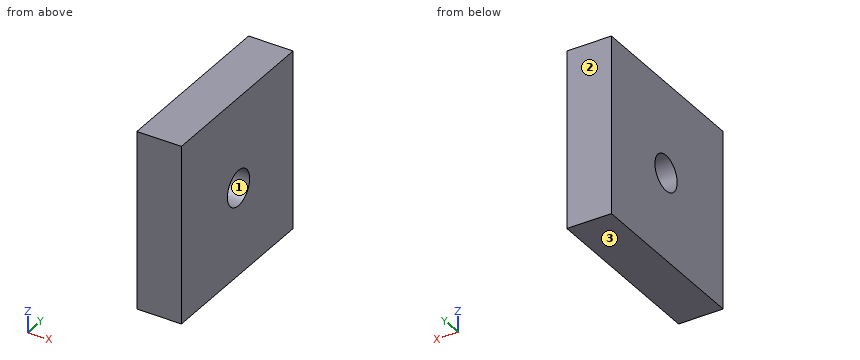
```python
from build123d import *

# Parameters (mm, degrees)
F0_W     = 25.4
F0_H     = 25.4
F1_DEPTH = 6.35
F2_R     = 2.52222
F3_DEPTH = 25.4


with BuildPart() as f1:
    # F0 (on Right) → F1 (new body)
    with BuildSketch(Plane.YZ):
        with Locations((12.7, 12.7)):
            Rectangle(F0_W, F0_H)
    extrude(amount=F1_DEPTH)

    # F2 (on face) → F3 (cut)
    with BuildSketch(Plane.YZ.offset(6.35)):
        with Locations((12.981366, 12.477624)):
            Circle(F2_R)
    extrude(amount=-F3_DEPTH, mode=Mode.SUBTRACT)


solid = f1.part
```
For this review, take the finished solid that the model builds, in its own axes (mm). Face numbers are marked on the shaded views. Round coordinates to 2 decimals unless told otherwise and drop trailing zeros. Loops run counter-clockwise (first coordinate to the right, second up) from the corner with the lowest first, then second, coordinate; pieces in that order, holes last.
(1) Wall thickness on line 1 along Z through (x, y) = (4.5, 14) (3 decimals); line 2 along Y through (x, z) = (4.25, 14.5); line 3 along Z through (x, y) = (2.25, 11): over which ranges is each line inside the solid? List them lowest first.
Returned:
line 1: z = 0 to 10.17, 14.785 to 25.4
line 2: y = 0 to 11.47, 14.49 to 25.4
line 3: z = 0 to 10.92, 14.04 to 25.4
(2) We need section A-A (x = 5.25). Give the boundary of the cut face in (y, z), plus the area to 3 significant figures.
Returned:
outline: (0, 0) - (25.4, 0) - (25.4, 25.4) - (0, 25.4) - close; hole circle Ø5.04 at (12.98, 12.48)
area: 625 mm2
(3) Mouldability with a two-part tool opening along Z and no side actions: class the marked faces 1, 2 and 3 as released by +Z, released by -Z, zero draft, split by the parting line, or undercut.
Returned:
face 1: undercut
face 2: zero draft
face 3: released by -Z
(4) Clearance check with a flat-ended pin moving along its axis: P1, Ø3, axis at y = 12.98, z = 12.48, coming from the -X side. State where the tip first meets the part, or that it passes through.
Returned:
P1: passes through
